Geometry check sheet. Reference: the model listing, model coordinates, mm. A direction names the side the tool comes from. Coordinates: 2 decimals unless noted, no trailing zeros. Loops run counter-clockwise (first coordinate to the right, second up) from the corner with the lowest first, then second, coordinate; pieces in that order, holes last.
from build123d import *

# Parameters (mm, degrees)
F0_W      = 50
F0_H      = 180
F1_DEPTH  = 8
F2_R      = 4
F3_DEPTH  = 5
F4_R      = 4
F5_DEPTH  = 5
F6_W      = 5
F6_H      = 15
F7_DEPTH  = 25
F8_R      = 2
F9_DEPTH  = 5
F10_R     = 2
F11_DEPTH = 5


with BuildPart() as f1:
    # F0 (on Top) → F1 (new body)
    with BuildSketch(Plane.XY):
        with Locations((-2.453425, -15.13525)):
            Rectangle(F0_W, F0_H)
    extrude(amount=-F1_DEPTH)

    # F2 (on face) → F3 (join)
    with BuildSketch(Plane(origin=(-27.453425, 0, 0), x_dir=(0, -1, 0), z_dir=(-1, 0, 0))):
        Polygon((-74.86475, 60), (-74.86475, 0), (105.13525, 0), (105.13525, 25), align=None)
        with Locations((-44.86475, 30)):
            Circle(F2_R, mode=Mode.SUBTRACT)
    extrude(amount=-F3_DEPTH)

    # F4 (on face) → F5 (join)
    with BuildSketch(Plane.YZ.offset(22.546575)):
        Polygon((-105.13525, 25), (-105.13525, 0), (74.86475, 0), (74.86475, 60), align=None)
        with Locations((44.86475, 30)):
            Circle(F4_R, mode=Mode.SUBTRACT)
    extrude(amount=-F5_DEPTH)

    # F6 (on face) → F7 (join)
    with BuildSketch(Plane.XY):
        with Locations((-14.953425, -82.021954)):
            Rectangle(F6_W, F6_H)
        with Locations((10.046575, -82.032483)):
            Rectangle(F6_W, F6_H)
    extrude(amount=F7_DEPTH)

    # F8 (on face) → F9 (cut)
    with BuildSketch(Plane.YZ.offset(-12.453425)):
        with Locations((-82.021954, 20)):
            Circle(F8_R)
    extrude(amount=-F9_DEPTH, mode=Mode.SUBTRACT)

    # F10 (on face) → F11 (cut)
    with BuildSketch(Plane(origin=(7.546575, 0, 0), x_dir=(0, -1, 0), z_dir=(-1, 0, 0))):
        with Locations((82.021954, 20)):
            Circle(F10_R)
    extrude(amount=-F11_DEPTH, mode=Mode.SUBTRACT)


solid = f1.part
1) Section check D-D on z = 43. Record the cut outline in (x, y), and give its area (3 significant figures).
Data:
outline: (-27.45, -12.56) - (-22.45, -12.56) - (-22.45, 74.86) - (-27.45, 74.86) - close; (17.55, -12.56) - (22.55, -12.56) - (22.55, 74.86) - (17.55, 74.86) - close
area: 874 mm2
2) Section check C-C on y = -63.5. Record the cut outline in (x, z).
Data:
outline: (-27.45, -8) - (22.55, -8) - (22.55, 33.1) - (17.55, 33.1) - (17.55, 0) - (-22.45, 0) - (-22.45, 33.1) - (-27.45, 33.1) - close
3) Material ranges on probe 1 along X at (y, z) = (55.5, 1.5); probe 2 along Z at (x, y) = (10, -35.5); probe 3 along Z at (x, y) = (18, -25), recorded low to high.
Data:
probe 1: x = -27.45 to -22.45, 17.55 to 22.55
probe 2: z = -8 to 0
probe 3: z = -8 to 40.58
4) Section check A-A on z = 8. Record the cut outline in (x, y), and give its area (3 significant figures).
Data:
outline: (-27.45, -105.14) - (-22.45, -105.14) - (-22.45, 74.86) - (-27.45, 74.86) - close; (-17.45, -89.52) - (-12.45, -89.52) - (-12.45, -74.52) - (-17.45, -74.52) - close; (7.55, -89.53) - (12.55, -89.53) - (12.55, -74.53) - (7.55, -74.53) - close; (17.55, -105.14) - (22.55, -105.14) - (22.55, 74.86) - (17.55, 74.86) - close
area: 1,950 mm2
5) Section check B-B on z = 20. Record the cut outline in (x, y).
Data:
outline: (-27.45, -105.14) - (-22.45, -105.14) - (-22.45, 74.86) - (-27.45, 74.86) - close; (-17.45, -89.52) - (-12.45, -89.52) - (-12.45, -84.02) - (-17.45, -84.02) - close; (-17.45, -80.02) - (-12.45, -80.02) - (-12.45, -74.52) - (-17.45, -74.52) - close; (7.55, -89.53) - (12.55, -89.53) - (12.55, -84.02) - (7.55, -84.02) - close; (7.55, -80.02) - (12.55, -80.02) - (12.55, -74.53) - (7.55, -74.53) - close; (17.55, -105.14) - (22.55, -105.14) - (22.55, 74.86) - (17.55, 74.86) - close
6) Depth check by flat-ended pin: pin 1 (5.5 mm diameter, centred on x = -14.5, y = -78.5, fed in from +Z); pin 2 (10 mm diameter, centred on x = -18, y = -33.5, fed in from +Z); pin 3 (2 mm diameter, centred on x = 8.5, y = -49, fed in from +Z). Enter the tip coordinate at first touch or a pass-through.
Data:
pin 1: stops at z = 25
pin 2: stops at z = 39.37
pin 3: stops at z = 0
7) Access from +Z, -Z, +X, -X, +Y, -Y to the whole of each face (thin tool, end or side, straight path). Record for faces 5 (the cylindrical face through (-14.92, -83.5, 21.35)), 6 (the flat face through (10, -74.532, 12)), 7 (the flat face through (-15, -82, 25)), 8 (the flat face through (10, -89.532, 12)).
Data:
face 5: none
face 6: +Z, +Y
face 7: +Z, +Y, -Y
face 8: +Z, -Y
8) Mould release check, pull along Z, two halves, no side actions. Record for faces 1 (the flat face through (22.547, -16, 19)), 2 (the flat face through (-3, -14, -8)), 3 (the cylindrical face through (20.08, 48.68, 31.2)), 4 (the cylindrical face through (-24.99, 41.05, 31.2)): +Z half, -Z half, draft (parallel to the pull), parting line (faces both ways), or undercut.
Data:
face 1: draft
face 2: -Z half
face 3: undercut
face 4: undercut
